Autodesk Inventor part; units mm, degrees
ref_plane "YZ Plane" through (0, 0, 0) normal (1, 0, 0) x (0, 1, 0)
ref_plane "XZ Plane" through (0, 0, 0) normal (0, 1, 0) x (-1, 0, 0)
ref_plane "XY Plane" through (0, 0, 0) normal (0, 0, 1) x (1, 0, 0)
sketch "Sketch1" plane through (0, 0, 0) normal (0, 1, 0) x (-1, 0, 0)
  line L0 (32.258, -22.4282) -> (-32.258, -22.4282)
  line L1 (-32.258, -22.4282) -> (-32.258, 22.4282)
  line L2 (-32.258, 22.4282) -> (32.258, 22.4282)
  line L3 (32.258, 22.4282) -> (32.258, -22.4282)
  circle A0 centre (6.858, -18.161) radius 1.5875
  circle A1 centre (6.858, 18.161) radius 1.5875
  line L4 (6.858, -18.161) -> (6.858, 18.161) construction
  point P0 (0, 0)
  point P1 (32.258, 0)
  point P2 (0, -22.4282)
  point P3 (6.858, 0)
  dimension "d0" = 64.516
  dimension "d1" = 44.8564
  dimension "d2" = 3.175
  dimension "d3" = 25.4
  dimension "d4" = 39.116
  dimension "d15" = 36.322
extrude "Extrusion1" add sketch "Sketch1" along normal blind 39.37
sketch "Sketch2" plane through (0, 39.37, 0) normal (0, 1, 0) x (1, 0, 0)
  line L0 (-24.1562, -22.4282) -> (-24.1562, 22.4282) construction
  line L1 (-24.1562, 22.4282) -> (-18.3585, 22.4282) construction
  line L2 (-18.3585, 22.4282) -> (-18.3585, -22.4282) construction
  line L3 (-18.3585, -22.4282) -> (-24.1562, -22.4282) construction
  line L4 (32.258, 22.4282) -> (-32.258, 22.4282)
  line L5 (-32.258, -22.4282) -> (32.258, -22.4282)
  point P0 (0, 0)
sketch "Sketch4" plane through (0, 0, 0) normal (0, -1, 0) x (1, 0, 0)
  circle A0 centre (-23.0124, -8.636) radius 3.175
  circle A1 centre (-23.0124, 8.636) radius 3.175
  line L0 (-32.258, -22.4282) -> (-32.258, 22.4282)
  circle A2 centre (-6.858, -18.161) radius 1.5875
  line L1 (-23.0124, -8.636) -> (-23.0124, 8.636) construction
  point P0 (0, 0)
  point P1 (-23.0124, 0)
  dimension "d11" = 17.272
  dimension "d12" = 9.2456
  dimension "d13" = 6.35
  dimension "d14" = 25.4
extrude "Extrusion2" add sketch "Sketch4" along normal blind 25.4 contours A0 | A1
properties part number "Pump"
Input: part model. Units: mm. Frame: model coordinates. A direction names the side the tool comes from. Round coordinates to 2 decimals unless told otherwise and drop trailing zeros. Loops run counter-clockwise (first coordinate to the right, second up) from the corner with the lowest first, then second, coordinate; pieces in that order, holes last.
1) Pin query (flat end, axial travel): pin 1 (1 mm diameter, centred on x = -0.5, z = 4.5, fed in from -Y); pin 2 (3 mm diameter, centred on y = -5.5, z = 4.5, fed in from -X); pin 3 (12 mm diameter, centred on y = -14.5, z = 11.5, fed in from -X); pin 4 (4 mm diameter, centred on x = -6.858, z = 18.161, fed in from +Y). Return the tip coordinate at first contact, or that it passes through.
Ans:
pin 1: stops at y = 0
pin 2: stops at x = -24.78
pin 3: stops at x = -26.19
pin 4: stops at y = 39.37
2) Section query A-A on z = -1. Return the cut outline in (x, y), plus the area to 3 significant figures.
Ans:
outline: (-32.26, 0) - (32.26, 0) - (32.26, 39.37) - (-32.26, 39.37) - close
area: 2,540 mm2
3) Pull-direction query (Z, two-part tool) for faces 1 (the flat face through (0, 19, 22.428)), 2 (the flat face through (-23, -25.4, 9)), 3 (the cylindrical face through (-26.184, -12.522, -8.776)); classes: released by +Z, released by -Z, zero draft, split by the parting line, or undercut.
Ans:
face 1: released by +Z
face 2: zero draft
face 3: undercut
4) Section query C-C on x = 3.5. Return the cut outline in (y, z), plus the area to 3 significant figures.
Ans:
outline: (0, -22.43) - (39.37, -22.43) - (39.37, 22.43) - (0, 22.43) - close
area: 1,770 mm2
5) Material intervals for line 1 (Z direction, x = -6.5, y = 17); line 2 (Y direction, x = 28, z = -3); line 3 (X direction, y = 30.5, z = 19.5), sorted ascending.
Ans:
line 1: z = -22.43 to -19.71, -16.61 to 16.61, 19.71 to 22.43
line 2: y = 0 to 39.37
line 3: x = -32.26 to -7.71, -6.01 to 32.26
6) Set-up query: faces 4 (the cylindrical face through (-26.184, -12.522, 8.496)), 5 (the flat face through (-32.258, 19, 0)). Return all of +Z, -Z, +X, -X, +Y, -Y with unobstructed straight access to the full face (end or side cutting, diameter ignored); none if empty.
Ans:
face 4: -Y
face 5: +Z, -Z, -X, +Y, -Y
7) Section query B-B on y = -18. Return the cut outline in (x, z) (3 decimals), plus the area to 3 significant figures.
Ans:
outline: circle Ø6.35 at (-23.012, -8.636); circle Ø6.35 at (-23.012, 8.636)
area: 63.3 mm2
